Part print with two shaded views. Sizes in mm from the minimum x, y, z corner. Give positions to 0.01 mm unless a question says otherwise; leave off trailing zeros. Order: outer loops, then holes, each group sorted by start corner. A loop starts at its lowest first (then second) coordinate and runs counter-clockwise, first axis right, second up. Notation, with made-up numbers: M 79.25,34 L 120.25,34 A22 cw 120.25,60 Z; hole C -6.5,57 d9. An arc over 180 degrees is marked long. Answer as CSV lines item,"result".
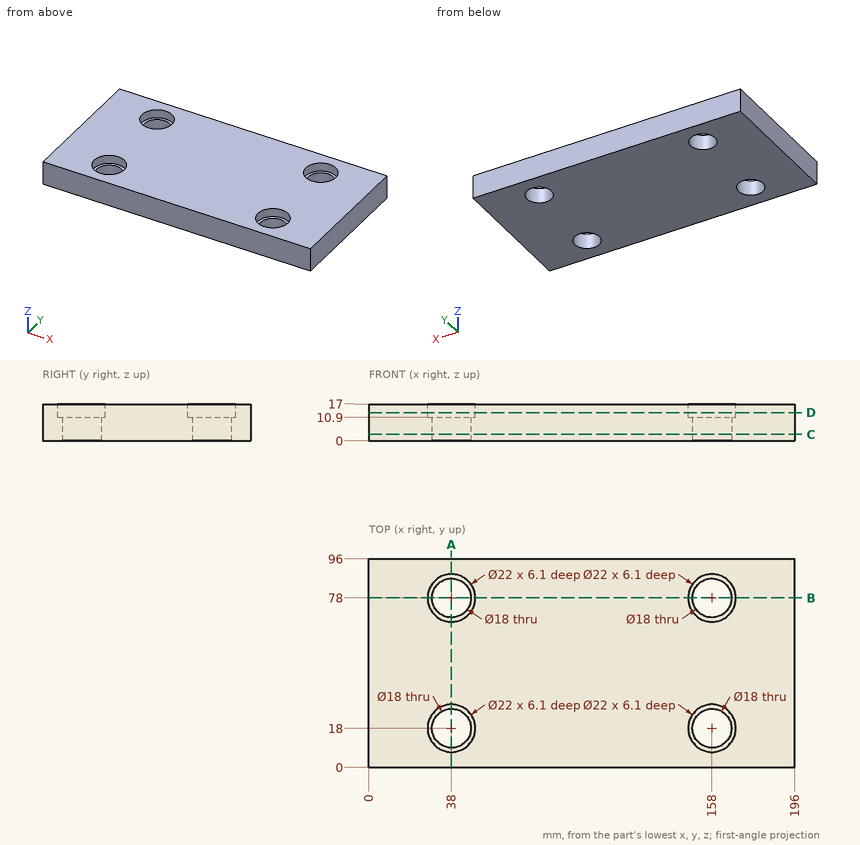
Item 1: Band-saw the part on A-A (x = 38). Give the cut face in (y, z).
Geometry says:
outline,"M 0,0 L 9,0 L 9,10.9 L 7,10.9 L 7,17 L 0,17 Z; M 27,0 L 69,0 L 69,10.9 L 67,10.9 L 67,17 L 29,17 L 29,10.9 L 27,10.9 Z; M 87,0 L 96,0 L 96,17 L 89,17 L 89,10.9 L 87,10.9 Z"
Item 2: Drop a flat-ended pin along its axis: pin 1 (20 mm diameter, centred on x = 158, y = 18, fed in from +Z). Give the stop position or say it passes through.
Geometry says:
pin 1,"stops at z = 10.9"
Item 3: Probe line 1 along Y through (x, z) = (158, 14.5); line 2 along X through (y, z) = (78.5, 11); line 3 along Y through (x, z) = (38, 5). List the from-to ranges inside material, lowest first. Write a range as from..to.
Geometry says:
line 1,"y = 0..7, 29..67, 89..96"
line 2,"x = 0..27.01, 48.99..147.01, 168.99..196"
line 3,"y = 0..9, 27..69, 87..96"
Item 4: Band-saw the part on C-C (z = 3). Give the cut face in (x, y).
Geometry says:
outline,"M 0,0 L 196,0 L 196,96 L 0,96 Z; hole C 38,18 d18; hole C 38,78 d18; hole C 158,18 d18; hole C 158,78 d18"
Item 5: Band-saw the part on B-B (y = 78). Give the cut face in (x, z).
Geometry says:
outline,"M 0,0 L 29,0 L 29,10.9 L 27,10.9 L 27,17 L 0,17 Z; M 47,0 L 149,0 L 149,10.9 L 147,10.9 L 147,17 L 49,17 L 49,10.9 L 47,10.9 Z; M 167,0 L 196,0 L 196,17 L 169,17 L 169,10.9 L 167,10.9 Z"
Item 6: Band-saw the part on D-D (z = 13). Give the cut face in (x, y), and give its area (3 significant figures).
Geometry says:
outline,"M 0,0 L 196,0 L 196,96 L 0,96 Z; hole C 38,18 d22; hole C 38,78 d22; hole C 158,18 d22; hole C 158,78 d22"
area,"17,300 mm2"
